from build123d import *

# Parameters (mm, degrees)
ESQUISSE1_W                           = 15
ESQUISSE1_H                           = 10
BOSS_EXTRU_1_DEPTH                    = 25
ENL_VEMENT_START                      = -6.2
ENL_VEMENT_DE_MATI_RE_BALAYAGE1_DEPTH = 6.2
ENL_V_MAT_EXTRU_1_REACH               = 32.822
ESQUISSE4_R                           = 1.75
ENL_V_MAT_EXTRU_2_REACH               = 32.822
ESQUISSE5_W                           = 2.7
ESQUISSE5_H                           = 5.9
ENL_V_MAT_EXTRU_3_REACH               = 32.822
ESQUISSE6_W                           = 5.9
ESQUISSE6_H                           = 2.7
ESQUISSE7_R                           = 1.75
ENL_V_MAT_EXTRU_4_DEPTH               = 8.5


# Read off the part's stored shape, not the designer's step: Enlèvement de matière-Balayage1
with BuildPart() as part:
    # Esquisse1 → Boss.-Extru.1 (new body)
    with BuildSketch(Plane(origin=(0, 0, 0), x_dir=(1, 0, 0), z_dir=(0, 1, 0))):
        with Locations((7.5, 5)):
            Rectangle(ESQUISSE1_W, ESQUISSE1_H)
    extrude(amount=BOSS_EXTRU_1_DEPTH)

    # Enlèvement de matière-Balayage1 outline → Enlèvement de matière-Balayage1 (cut)
    with BuildSketch(Plane.XY.offset(ENL_VEMENT_START)):
        with BuildLine():
            Line((10.8, 25), (10.8, 18.967282711))
            ThreePointArc((10.8, 18.967282711), (10.254975604, 17.150662382), (8.799933685, 15.934104112))
            Line((8.799933685, 15.934104112), (7.254659998, 15.27184396))
            ThreePointArc((7.254659998, 15.27184396), (4.741405774, 13.170516039), (3.8, 10.032717289))
            Line((3.8, 10.032717289), (3.8, 9.348137929))
            ThreePointArc((3.8, 9.348137929), (4.926930309, 5.94563391), (7.862117052, 3.888528103))
            Line((7.862117052, 3.888528103), (15, 1.747163219))
            Line((15, 1.747163219), (15, 3.41761226))
            Line((15, 3.41761226), (8.321873669, 5.42105016))
            ThreePointArc((8.321873669, 5.42105016), (6.210598994, 6.900722757), (5.4, 9.348137929))
            Line((5.4, 9.348137929), (5.4, 10.032717289))
            ThreePointArc((5.4, 10.032717289), (6.077151522, 12.289730425), (7.884930876, 13.801211912))
            Line((7.884930876, 13.801211912), (9.430204563, 14.463472064))
            ThreePointArc((9.430204563, 14.463472064), (11.590721352, 16.269876768), (12.4, 18.967282711))
            Line((12.4, 18.967282711), (12.4, 25))
            Line((12.4, 25), (10.8, 25))
        make_face()
    extrude(amount=ENL_VEMENT_DE_MATI_RE_BALAYAGE1_DEPTH, mode=Mode.SUBTRACT)

    # Esquisse4 → Enlèv. mat.-Extru.1 (cut, up to next)
    with BuildSketch(Plane(origin=(15, 0, 0), x_dir=(0, 0, -1), z_dir=(1, 0, 0)), mode=Mode.PRIVATE) as enl_v_mat_extru_1_sk1:
        with Locations((3.1, 9.5)):
            Circle(ESQUISSE4_R)
    enl_v_mat_extru_1_tool1 = extrude(enl_v_mat_extru_1_sk1.sketch, amount=-ENL_V_MAT_EXTRU_1_REACH, mode=Mode.PRIVATE) & part.part
    add(enl_v_mat_extru_1_tool1.solids().sort_by_distance((15, 9.5, -3.1))[0], mode=Mode.SUBTRACT)

    # Esquisse5 → Enlèv. mat.-Extru.2 (cut, up to next)
    with BuildSketch(Plane.XY, mode=Mode.PRIVATE) as enl_v_mat_extru_2_sk1:
        with Locations((11.15, 9.5)):
            Rectangle(ESQUISSE5_W, ESQUISSE5_H)
    enl_v_mat_extru_2_tool1 = extrude(enl_v_mat_extru_2_sk1.sketch, amount=-ENL_V_MAT_EXTRU_2_REACH, mode=Mode.PRIVATE) & part.part
    add(enl_v_mat_extru_2_tool1.solids().sort_by_distance((11.15, 9.5, 0))[0], mode=Mode.SUBTRACT)

    # Symétrie1: part across plane


with BuildPart() as part_1:
    add(part.part)
    add(part.part.mirror(Plane(origin=(0, 0, 0), x_dir=(0, 0, 1), z_dir=(0, -1, 0))))

    # Esquisse6 → Enlèv. mat.-Extru.3 (cut, up to next)
    with BuildSketch(Plane.XY, mode=Mode.PRIVATE) as enl_v_mat_extru_3_sk1:
        with Locations((5.4, -21.15)):
            Rectangle(ESQUISSE6_W, ESQUISSE6_H)
    enl_v_mat_extru_3_tool1 = extrude(enl_v_mat_extru_3_sk1.sketch, amount=-ENL_V_MAT_EXTRU_3_REACH, mode=Mode.PRIVATE) & part_1.part
    add(enl_v_mat_extru_3_tool1.solids().sort_by_distance((5.4, -21.15, 0))[0], mode=Mode.SUBTRACT)

    # Esquisse7 → Enlèv. mat.-Extru.4 (cut)
    with BuildSketch(Plane.XZ.offset(25)):
        with Locations(Location((5.4, -5, 0), (0, 0, 270))):
            Circle(ESQUISSE7_R)
    extrude(amount=-ENL_V_MAT_EXTRU_4_DEPTH, mode=Mode.SUBTRACT)


solid = part_1.part
For this review, take the finished solid that the model builds, in its own axes (mm). A direction names the side the tool comes from. Coordinates: 2 decimals unless noted, no trailing zeros. Order: outer loops, then holes, each group sorted by start corner. A loop starts at its lowest first (then second) coordinate and runs counter-clockwise, first axis right, second up. Notation, with made-up numbers: (-1, 16) -> (41, 16) arc R20 ccw to (41, 26) -> close; hole circle Ø5 at (41.5, 6). An arc over 180 degrees is marked (long way). Return JSON: item names as keys, results as strings.
1. For pin 1 Ø0.8 at (y, z) = (10, -2) entering from +X, flat-tipped, find the tip position at first contact; note if it passes through.
Answer block:
{"pin 1": "x = 3.81"}
2. The part is to be moulded in two halves that separate along X. For faces 1 (the cylindrical face through (13.768, -11.235, -2.872)), 2 (the cylindrical face through (6.06, -12.26, -3.14)), say which applies: +X half, -X half, draft (parallel to the pull), parting line (faces both ways), or undercut.
Answer block:
{"face 1": "draft", "face 2": "undercut"}
3. We need section A-A on x = 3. Write out the cut boundary in (y, z).
Answer block:
{"outline": "(-25, -10) -> (-22.5, -10) -> (-22.5, 0) -> (-25, 0) -> close; (-19.8, -10) -> (25, -10) -> (25, 0) -> (-19.8, 0) -> close"}
4. We need section C-C on x = 14. Write out the cut boundary in (y, z), and give its area (3 significant figures).
Answer block:
{"outline": "(-25, -10) -> (25, -10) -> (25, 0) -> (3.72, 0) -> (3.72, -6.2) -> (2.05, -6.2) -> (2.05, 0) -> (-2.05, 0) -> (-2.05, -6.2) -> (-3.72, -6.2) -> (-3.72, 0) -> (-25, 0) -> close; hole circle Ø3.5 at (-9.5, -3.1); hole circle Ø3.5 at (9.5, -3.1)", "area": "460 mm²"}
5. For line 1 (X direction, y = -22, z = -5); line 2 (X direction, y = -20, z = -7); line 3 (X direction, y = -19, z = -5), list the stretches that pass through material, from the lowest coordinate up. Write a range as from..to.
Answer block:
{"line 1": "0..2.45, 8.35..10.8, 12.4..15", "line 2": "0..2.45, 8.35..15", "line 3": "0..3.65, 7.15..10.8, 12.4..15"}
6. Machinability: for faces 3 (the cylindrical face through (4.77, -13.21, -3.14)), 4 (the flat face through (12.4, 22, -3)), 5 (the flat face through (3, -22.5, -5)), which of the approach directions +Z, -Z, +X, -X, +Y, -Y give a long, thin tool a straight path to every point of the face, cutting with its end or side? Answer none if there is none.
Answer block:
{"face 3": "+Z", "face 4": "+Z, +Y", "face 5": "+Z, -Z"}
7. We need section B-B on z = -5.5. State how many separate pieces and enclosed holes the cut face has, and give its area (3 significant figures).
Answer block:
{"separate pieces": "3", "enclosed holes": "2", "area": "579 mm²"}
